Part model, mm, in its own coordinate system. Round coordinates to 2 decimals unless told otherwise and drop trailing zeros. Loops run counter-clockwise (first coordinate to the right, second up) from the corner with the lowest first, then second, coordinate; pieces in that order, holes last. Notation, with made-up numbers: (-28.5, 3) - (-8.5, 3) arc R17 cw to (-8.5, 10) - close; hole circle Ø10 at (44.5, 50). An arc over 180 degrees is marked (long way). Write each question's results on one line, items separated by ' | '. Start each with the question number.
(1) Cut at B-B, the plane y = 1.5. List the corners of the cut face in (x, z).
(2) Flat gauge pins, fed straight in: P1, Ø11, axis at x = -37.13, y = -21.44, coming from the -Z side; P2, Ø5, axis at x = -34.5, z = -5, coming from the -Y side; P3, Ø8, axis at y = 8.5, z = 1, coming from the -X side; P4, Ø4, axis at y = -4, z = 4, coming from the -X side. Where does each tip first touch, or does it go through?
(3) Drill centre lines: L1, parallel to Y at x = 0, z = 0.25; L2, parallel to X at y = -2, z = 6; L3, parallel to Y at x = 34.5, z = 2.5. Where is each one in solid material? Low to high.
(4) Cut at A-A, the plane x = 0. List the corners of the cut face in (y, z).
(5) Mould opens along Y. For faces 1 (the face through (-1, -11, -7.112)), 2 (the face through (-11.012, -49.592, 0.1)), 3 (the face through (-41.89, -21.23, 0.1)), 4 (the face through (10.86, -1.46, -1.15)) say: released by +Y, released by -Y, zero draft, split by the parting line, or undercut.
(6) Cut at D-D, the plane z = 2.5. Give the number of separate pieces and of enclosed holes in the cut face, then the cut area to 3 significant figures.
(7) Cut at C-C, the plane x = 36.5. List the corners of the cut face in (y, z), then the cut area to 3 significant figures.
from build123d import *

# Parameters (mm, degrees)
SKETCH1_R           = 50.8
BOSS_EXTRUDE1_DEPTH = 7.112
SKETCH2_R           = 5.55625
CUT_EXTRUDE1_DEPTH  = 74.236617726
SKETCH3_R           = 4.7625
CUT_EXTRUDE2_DEPTH  = 74.236617726
CIRPATTERN1_COUNT   = 6
SKETCH5_R           = 4.8768
CUT_EXTRUDE3_DEPTH  = 25.4


with BuildPart() as part:
    # Sketch1 → Boss-Extrude1 (new, symmetric)
    with BuildSketch(Plane.XY):
        Circle(SKETCH1_R)
    extrude(amount=BOSS_EXTRUDE1_DEPTH, both=True)

    # Sketch2 → Cut-Extrude1 (cut, through all)
    with BuildSketch(Plane.XY.offset(7.112)):
        Circle(SKETCH2_R)
    extrude(amount=-CUT_EXTRUDE1_DEPTH, mode=Mode.SUBTRACT)

    # Sketch3 → Cut-Extrude2 (cut, through all)
    with BuildSketch(Plane.XY.offset(7.112)):
        with Locations((0, 42.8752)):
            Circle(SKETCH3_R)
    cut_extrude2 = extrude(amount=-CUT_EXTRUDE2_DEPTH, mode=Mode.SUBTRACT)

    # CirPattern1: Cut-Extrude2 ×6 about axis
    cirpattern1_axis = Axis((0, 0, 0), (0, 0, 1))
    for i in range(1, CIRPATTERN1_COUNT):
        add(cut_extrude2.rotate(cirpattern1_axis, i * 360 / CIRPATTERN1_COUNT), mode=Mode.SUBTRACT)

    # Sketch5 → Cut-Extrude3 (cut, symmetric)
    with BuildSketch(Plane(origin=(-0.876216993, 0, 3.270086336), x_dir=(0, -1, 0), z_dir=(-0.25881904510252135, 0, 0.9659258262890681))):
        with Locations(Location((0, 14.844014522, 0), (0, 0, 270))):
            Circle(SKETCH5_R)
    extrude(amount=CUT_EXTRUDE3_DEPTH, both=True, mode=Mode.SUBTRACT)


solid = part.part
A:
1) outline: (-50.78, -7.11) - (-5.35, -7.11) - (-5.35, 7.11) - (-50.78, 7.11) - close; (5.35, -7.11) - (12.47, -7.11) - (8.66, 7.11) - (5.35, 7.11) - close; (18.27, 7.11) - (22.08, -7.11) - (50.78, -7.11) - (50.78, 7.11) - close
2) P1: z = -7.11 | P2: y = -39.45 | P3: x = -50.6 | P4: x = -50.76
3) L1: -50.8 to -47.64, -38.11 to -5.56, 5.56 to 38.11, 47.64 to 50.8 | L2: -50.76 to -5.18, 5.18 to 9.16, 18.36 to 50.76 | L3: -37.29 to -25.41, -17.47 to 17.47, 25.41 to 37.29
4) outline: (-50.8, -7.11) - (-47.64, -7.11) - (-47.64, 7.11) - (-50.8, 7.11) - close; (-38.11, -7.11) - (-5.56, -7.11) - (-5.56, 7.11) - (-38.11, 7.11) - close; (5.56, -7.11) - (38.11, -7.11) - (38.11, 7.11) - (5.56, 7.11) - close; (47.64, -7.11) - (50.8, -7.11) - (50.8, 7.11) - (47.64, 7.11) - close
5) face 1: zero draft | face 2: split by the parting line | face 3: undercut | face 4: undercut
6) separate pieces: 1 | enclosed holes: 8 | area: 7,510 mm2
7) outline: (-35.33, -7.11) - (-26.16, -7.11) - (-26.16, 7.11) - (-35.33, 7.11) - close; (-16.72, -7.11) - (16.72, -7.11) - (16.72, 7.11) - (-16.72, 7.11) - close; (26.16, -7.11) - (35.33, -7.11) - (35.33, 7.11) - (26.16, 7.11) - close | area: 737 mm2
